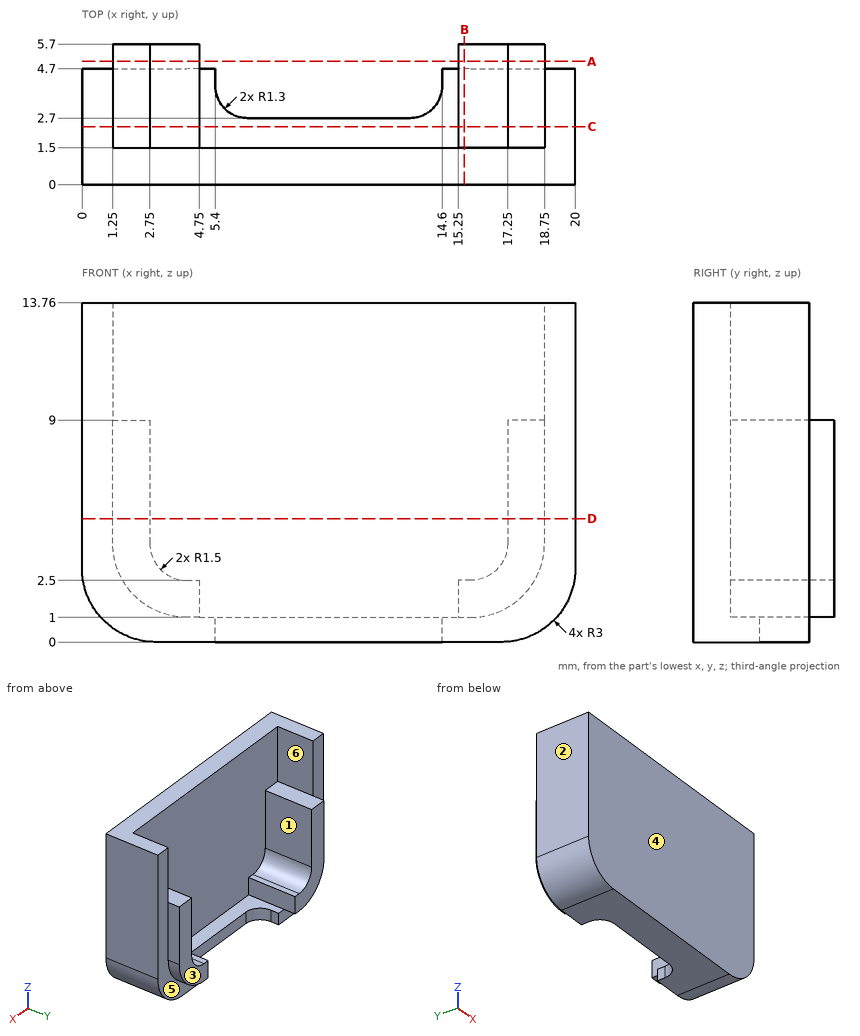
Drawing for the job (mm, zero at the part's lowest x, y, z). A direction names the side the tool comes from. Give positions to 0.01 mm unless a question says otherwise; leave off trailing zeros. Loops run counter-clockwise (first coordinate to the right, second up) from the corner with the lowest first, then second, coordinate; pieces in that order, holes last.
(1) 3-axis set-ups, long thin cutter, end or side, ignore diameter. For the marked faces 4, 5 and 6: which of +Z, -Z, +X, -X, +Y, -Y reach the whole face in a straight line?
Return value:
face 4: +Z, -Z, +X, -X, -Y
face 5: -Z, +X, +Y
face 6: +Z, +Y
(2) Band-saw the part on B-B (x = 15.5). Write the cut outline in (y, z).
Return value:
outline: (0, 0) - (4.7, 0) - (4.7, 1) - (5.7, 1) - (5.7, 2.5) - (1.5, 2.5) - (1.5, 13.76) - (0, 13.76) - close
(3) Band-saw the part on D-D (z = 5). Write the cut outline in (x, y), and give its area (3 significant figures).
Return value:
outline: (0, 0) - (20, 0) - (20, 4.7) - (18.75, 4.7) - (18.75, 5.7) - (17.25, 5.7) - (17.25, 1.5) - (2.75, 1.5) - (2.75, 5.7) - (1.25, 5.7) - (1.25, 4.7) - (0, 4.7) - close
area: 50.6 mm2
(4) Pin check, flat tips, straight feed: pin 1 (2 mm diameter, centred on x = 6, z = 3.5, fed in from +Y); pin 2 (0.8 mm diameter, centred on x = 9, z = 0.5, fed in from +Y); pin 3 (0.8 mm diameter, centred on y = 4, z = 1.5, fed in from +X). Stop position of each tip, or through.
Return value:
pin 1: stops at y = 1.5
pin 2: stops at y = 2.7
pin 3: stops at x = 19.79
(5) Band-saw the part on C-C (y = 2.35). Write the cut outline in (x, z).
Return value:
outline: (0, 3) arc R3 ccw to (3, 0) - (17, 0) arc R3 ccw to (20, 3) - (20, 13.76) - (18.75, 13.76) - (18.75, 9) - (17.25, 9) - (17.25, 4) arc R1.5 cw to (15.75, 2.5) - (15.25, 2.5) - (15.25, 1) - (4.75, 1) - (4.75, 2.5) - (4.25, 2.5) arc R1.5 cw to (2.75, 4) - (2.75, 9) - (1.25, 9) - (1.25, 13.76) - (0, 13.76) - close
(6) Band-saw the part on A-A (y = 5). Write the cut outline in (x, z).
Return value:
outline: (1.25, 4) arc R3 ccw to (4.25, 1) - (4.75, 1) - (4.75, 2.5) - (4.25, 2.5) arc R1.5 cw to (2.75, 4) - (2.75, 9) - (1.25, 9) - close; (15.25, 1) - (15.75, 1) arc R3 ccw to (18.75, 4) - (18.75, 9) - (17.25, 9) - (17.25, 4) arc R1.5 cw to (15.75, 2.5) - (15.25, 2.5) - close
(7) Drill centre lines: line 1 along X through (y, z) = (2.65, 10); line 2 along X through (y, z) = (2.8, 5); line 3 along Z through (x, y) = (5.75, 2.85). Where is each one in solid material? Low to high.
Return value:
line 1: x = 0 to 1.25, 18.75 to 20
line 2: x = 0 to 2.75, 17.25 to 20
line 3: z = 0 to 1
(8) Pull direction X, two halves, no side cores. Call the marked faces 1, 2 and 3: pulls with the +X half, pulls with the -X half, needs draft (parallel to the pull), parting line crosses it, or undercut.
Return value:
face 1: undercut
face 2: pulls with the -X half
face 3: needs draft
